Source: CAD feature listing. Evaluate the final solid. Frame: model axes, mm. A direction names the side the tool comes from. Coordinates: 2 decimals unless noted, no trailing zeros. Write each loop counter-clockwise with the first axis right and the second up, starting at its lowest first coordinate (ties: lowest second). Pieces come first, ordered by that corner, then holes. Notation, with made-up numbers: (57, -19) - (95, -19) arc R5 cw to (95, -13) - close; hole circle Ø5 at (1, 42). An arc over 180 degrees is marked (long way). One line per question, with ' | ' between items.
from build123d import *

# Parameters (mm, degrees)
ESQUISSE1_W              = 40
ESQUISSE1_H              = 40
BOSS_EXTRU_1_DEPTH       = 50
ESQUISSE2_R              = 5
ENL_V_MAT_EXTRU_1_DEPTH  = 41
ESQUISSE3_R              = 5
ENL_V_MAT_EXTRU_2_DEPTH  = 41
ESQUISSE4_W              = 20
ESQUISSE4_H              = 14
ENL_V_MAT_EXTRU_3_DEPTH  = 29
ESQUISSE5_W              = 14
ESQUISSE5_H              = 20
ENL_V_MAT_EXTRU_4_DEPTH  = 29
ESQUISSE6_W              = 22
ESQUISSE6_H              = 14
ENL_V_MAT_EXTRU_5_DEPTH  = 24
ESQUISSE7_W              = 14
ESQUISSE7_H              = 22
ENL_V_MAT_EXTRU_6_DEPTH  = 24
ESQUISSE8_R              = 11
ENL_V_MAT_EXTRU_7_DEPTH  = 7
ESQUISSE9_R              = 12.5
ENL_V_MAT_EXTRU_8_DEPTH  = 1.5
ESQUISSE10_R             = 11
ENL_V_MAT_EXTRU_9_DEPTH  = 7
ESQUISSE11_R             = 12.5
ENL_V_MAT_EXTRU_10_DEPTH = 1.5
ESQUISSE12_W             = 40
ESQUISSE12_H             = 40
BOSS_EXTRU_2_DEPTH       = 7
ESQUISSE13_R             = 2.25
ENL_V_MAT_EXTRU_11_DEPTH = 15
ESQUISSE14_W             = 3
ESQUISSE14_H             = 7
ENL_V_MAT_EXTRU_12_DEPTH = 12
ESQUISSE15_W             = 7
ESQUISSE15_H             = 3
ENL_V_MAT_EXTRU_13_DEPTH = 12


with BuildPart() as part:
    # Esquisse1 → Boss.-Extru.1 (new body)
    with BuildSketch(Plane.XY):
        with Locations((-20, 20)):
            Rectangle(ESQUISSE1_W, ESQUISSE1_H)
    extrude(amount=BOSS_EXTRU_1_DEPTH)

    # Esquisse2 → Enlèv. mat.-Extru.1 (cut, through all)
    with BuildSketch(Plane(origin=(0, 40, 0), x_dir=(1, 0, 0), z_dir=(0, 1, 0))):
        with Locations(Location((-20, -15, 0), (0, 0, 270))):  # turned: the seam where the file's is
            Circle(ESQUISSE2_R)
    extrude(amount=-ENL_V_MAT_EXTRU_1_DEPTH, mode=Mode.SUBTRACT)

    # Esquisse3 → Enlèv. mat.-Extru.2 (cut, through all)
    with BuildSketch(Plane.ZY.offset(40)):
        with Locations((35, 20)):
            Circle(ESQUISSE3_R)
    extrude(amount=-ENL_V_MAT_EXTRU_2_DEPTH, mode=Mode.SUBTRACT)

    # Esquisse4 → Enlèv. mat.-Extru.3 (cut)
    with BuildSketch(Plane.ZY.offset(40)):
        with Locations((15, 20)):
            Rectangle(ESQUISSE4_W, ESQUISSE4_H)
    extrude(amount=-ENL_V_MAT_EXTRU_3_DEPTH, mode=Mode.SUBTRACT)

    # Esquisse5 → Enlèv. mat.-Extru.4 (cut)
    with BuildSketch(Plane.XZ):
        with Locations((-20, 35)):
            Rectangle(ESQUISSE5_W, ESQUISSE5_H)
    extrude(amount=-ENL_V_MAT_EXTRU_4_DEPTH, mode=Mode.SUBTRACT)

    # Esquisse6 → Enlèv. mat.-Extru.5 (cut)
    with BuildSketch(Plane(origin=(0, 0, 0), x_dir=(0, 0, -1), z_dir=(1, 0, 0))):
        with Locations((-11, 20)):
            Rectangle(ESQUISSE6_W, ESQUISSE6_H)
    extrude(amount=-ENL_V_MAT_EXTRU_5_DEPTH, mode=Mode.SUBTRACT)

    # Esquisse7 → Enlèv. mat.-Extru.6 (cut)
    with BuildSketch(Plane(origin=(0, 40, 0), x_dir=(1, 0, 0), z_dir=(0, 1, 0))):
        with Locations((-20, -39)):
            Rectangle(ESQUISSE7_W, ESQUISSE7_H)
    extrude(amount=-ENL_V_MAT_EXTRU_6_DEPTH, mode=Mode.SUBTRACT)

    # Esquisse8 → Enlèv. mat.-Extru.7 (cut)
    with BuildSketch(Plane(origin=(0, 0, 0), x_dir=(0, 0, -1), z_dir=(1, 0, 0))):
        with Locations(Location((-35, 20, 0), (0, 0, 90))):  # turned: the seam where the file's is
            Circle(ESQUISSE8_R)
    extrude(amount=-ENL_V_MAT_EXTRU_7_DEPTH, mode=Mode.SUBTRACT)

    # Esquisse9 → Enlèv. mat.-Extru.8 (cut)
    with BuildSketch(Plane(origin=(0, 0, 0), x_dir=(0, 0, -1), z_dir=(1, 0, 0))):
        with Locations(Location((-35, 20, 0), (0, 0, 90))):  # turned: the seam where the file's is
            Circle(ESQUISSE9_R)
    extrude(amount=-ENL_V_MAT_EXTRU_8_DEPTH, mode=Mode.SUBTRACT)

    # Esquisse10 → Enlèv. mat.-Extru.9 (cut)
    with BuildSketch(Plane(origin=(0, 40, 0), x_dir=(1, 0, 0), z_dir=(0, 1, 0))):
        with Locations(Location((-20, -15, 0), (0, 0, 270))):  # turned: the seam where the file's is
            Circle(ESQUISSE10_R)
    extrude(amount=-ENL_V_MAT_EXTRU_9_DEPTH, mode=Mode.SUBTRACT)

    # Esquisse11 → Enlèv. mat.-Extru.10 (cut)
    with BuildSketch(Plane(origin=(0, 40, 0), x_dir=(1, 0, 0), z_dir=(0, 1, 0))):
        with Locations(Location((-20, -15, 0), (0, 0, 270))):  # turned: the seam where the file's is
            Circle(ESQUISSE11_R)
    extrude(amount=-ENL_V_MAT_EXTRU_10_DEPTH, mode=Mode.SUBTRACT)

    # Esquisse12 → Boss.-Extru.2 (add)
    with BuildSketch(Plane(origin=(0, 0, 0), x_dir=(-1, 0, 0), z_dir=(0, 0, -1))):
        with Locations((20, 20)):
            Rectangle(ESQUISSE12_W, ESQUISSE12_H)
    extrude(amount=BOSS_EXTRU_2_DEPTH)

    # Esquisse13 → Enlèv. mat.-Extru.11 (cut)
    with BuildSketch(Plane(origin=(0, 0, -7), x_dir=(-1, 0, 0), z_dir=(0, 0, -1))):
        with Locations((10, 7.5)):
            Circle(ESQUISSE13_R)
        with Locations((32.5, 30)):
            Circle(ESQUISSE13_R)
    extrude(amount=-ENL_V_MAT_EXTRU_11_DEPTH, mode=Mode.SUBTRACT)

    # Esquisse14 → Enlèv. mat.-Extru.12 (cut)
    with BuildSketch(Plane.ZY.offset(40)):
        with Locations((-1.5, 30)):
            Rectangle(ESQUISSE14_W, ESQUISSE14_H)
    extrude(amount=-ENL_V_MAT_EXTRU_12_DEPTH, mode=Mode.SUBTRACT)

    # Esquisse15 → Enlèv. mat.-Extru.13 (cut)
    with BuildSketch(Plane.XZ):
        with Locations((-10, -1.5)):
            Rectangle(ESQUISSE15_W, ESQUISSE15_H)
    extrude(amount=-ENL_V_MAT_EXTRU_13_DEPTH, mode=Mode.SUBTRACT)


solid = part.part
Item 1: Cut plane B-B on x = -22. State how many separate pieces and enclosed holes the cut face has, and give its area (3 significant figures).
Check sheet entries:
separate pieces: 4 | enclosed holes: 0 | area: 713 mm²
Item 2: Mould query, pull axis Y, two halves, no side actions, for faces 6 (the face through (-12, 20, 0)), 7 (the face through (-35, 30, -3)), 8 (the face through (-20, 0, 22)), 9 (the face through (-24.436, 30.042, 17.307)). Classes: pulls with the +Y half, pulls with the -Y half, needs draft (parallel to the pull), parting line crosses it, or undercut.
Check sheet entries:
face 6: undercut | face 7: undercut | face 8: pulls with the -Y half | face 9: needs draft
Item 3: Cut plane A-A on z = 35. Return loops of the section in (x, y), and give its area (4 significant figures).
Check sheet entries:
outline: (-40, 0) - (-27, 0) - (-27, 15) - (-40, 15) - close; (-40, 25) - (-27, 25) - (-27, 40) - (-40, 40) - close; (-13, 0) - (0, 0) - (0, 7.5) - (-1.5, 7.5) - (-1.5, 9) - (-7, 9) - (-7, 15) - (-13, 15) - close; (-13, 25) - (-7, 25) - (-7, 31) - (-1.5, 31) - (-1.5, 32.5) - (0, 32.5) - (0, 40) - (-13, 40) - close | area: 691.5 mm²
Item 4: Pin query (flat end, axial travel): pin 1 Ø1.5 at (x, z) = (-24.5, 29) entering from -Y; pin 2 Ø12.5 at (x, z) = (-19, 10.5) entering from +Y; pin 3 Ø3.5 at (x, y) = (-32.5, 30) entering from -Z; pin 4 Ø1.5 at (x, z) = (-8.5, -2) entering from -Y. Return the tip coordinate at first contact, or that it passes through.
Check sheet entries:
pin 1: through | pin 2: y = 33 | pin 3: z = 8 | pin 4: y = 12
Item 5: Cut plane D-D on y = 14. Return loops of the section in (x, z).
Check sheet entries:
outline: (-40, -7) - (0, -7) - (0, 0) - (-24, 0) - (-24, 5) - (-40, 5) - close; (-40, 25) - (-27, 25) - (-27, 45) - (-13, 45) - (-13, 25) - (-11, 25) - (-11, 22) - (0, 22) - (0, 24.03) - (-1.5, 24.03) - (-1.5, 25.78) - (-7, 25.78) - (-7, 44.22) - (-1.5, 44.22) - (-1.5, 45.97) - (0, 45.97) - (0, 50) - (-40, 50) - close
Item 6: Ray query, line 1 along Y through (x, z) = (-10, 3.25); line 2 along Y through (x, z) = (-31, 35); line 3 along Y through (x, z) = (-13, 24). Return the intervals inside material, ascending. Write a range as [from, to].
Check sheet entries:
line 1: [0, 5.25], [9.75, 13], [27, 40] | line 2: [0, 15], [25, 40] | line 3: [0, 13], [27, 38.5]
Item 7: Access query for faces 1 (the face through (-20, 35, 28)), 2 (the face through (-34, 20, 25)), 3 (the face through (-20, 6, 25)), 4 (the face through (-24, 20, 3)), 5 (the face through (-22, 33, 20)). Directions: +Z, -Z, +X, -X, +Y, -Y. A direction counts if a zero-diameter tool reaches every point of the face in a straight line with its end or side. Return the directions, or none.
Check sheet entries:
face 1: +Z, +Y, -Y | face 2: -X | face 3: -Y | face 4: +X | face 5: +Y
